Autodesk Inventor part; units mm, degrees
ref_plane "Work Plane1" through (0, 58, 0) normal (0, 1, 0) x (1, 0, 0)
ref_plane "YZ Plane" through (0, 0, 0) normal (1, 0, 0) x (0, 1, 0)
ref_plane "XZ Plane" through (0, 0, 0) normal (0, 1, 0) x (-1, 0, 0)
sketch "Sketch1" plane through (0, 0, 0) normal (0, 1, 0) x (-1, 0, 0)
  line L0 (25, 35) -> (-25, 35)
  line L1 (-25, 35) -> (-25, -35)
  line L2 (-25, -35) -> (25, -35)
  line L3 (25, -35) -> (25, 35)
  line L4 (25, 35) -> (-25, -35) construction
  line L5 (-25, 35) -> (25, -35) construction
  point P0 (0, 0)
  dimension "d0" = 50
  dimension "d1" = 70
extrude "Extrusion1" add sketch "Sketch1" along normal blind 4
sketch "Sketch2" plane through (0, 4, 0) normal (0, 1, 0) x (1, 0, 0)
  line L0 (25, -35) -> (25, 35)
  line L1 (25, 35) -> (-25, 35)
  line L2 (25, -35) -> (20, -35)
  line L3 (20, -35) -> (20, 35)
  line L4 (20, 35) -> (25, 35)
  line L5 (25, 35) -> (25, -35)
  line L6 (-25, 35) -> (-25, -35)
  line L7 (-25, -35) -> (-20, -35)
  line L8 (-20, -35) -> (-20, 35)
  line L9 (-20, 35) -> (-25, 35)
  line L10 (-25, 35) -> (-25, -35)
  point P0 (0, 0)
  dimension "d4" = 5
  dimension "d5" = 5
  dimension "d6" = 70
extrude "Extrusion2" add sketch "Sketch2" along normal blind 20
sketch "Sketch3" plane through (0, 24, 0) normal (0, 1, 0) x (1, 0, 0)
  line L0 (-25, -35) -> (25, -35)
  line L1 (25, -35) -> (25, 35)
  line L2 (-25, -35) -> (25, -35)
  line L3 (25, -35) -> (25, 35)
  line L4 (25, 35) -> (-25, 35)
  line L5 (-25, 35) -> (-25, -35)
  line L6 (-20, -20) -> (20, -20)
  line L7 (20, -20) -> (20, 20)
  line L8 (20, 20) -> (-20, 20)
  line L9 (-20, 20) -> (-20, -20)
  line L10 (-20, -20) -> (20, 20) construction
  line L11 (20, -20) -> (-20, 20) construction
  line L12 (-15.5, -29) -> (7.5, -29) construction
  line L13 (7.5, -29) -> (7.5, 29) construction
  line L14 (7.5, 29) -> (-15.5, 29) construction
  line L15 (-15.5, 29) -> (-15.5, -29) construction
  circle A0 centre (-15.5, -29) radius 1.5
  circle A1 centre (-15.5, 29) radius 1.5
  circle A2 centre (7.5, 29) radius 1.5
  circle A3 centre (7.5, -29) radius 1.5
  point P0 (0, 0)
  dimension "d9" = 40
  dimension "d10" = 40
  dimension "d13" = 23
  dimension "d14" = 58
  dimension "d15" = 6
  dimension "d16" = 4.5
  dimension "d17" = 3
  dimension "d18" = 3
  dimension "d19" = 3
  dimension "d20" = 3
extrude "Extrusion3" add sketch "Sketch3" along normal blind 4
sketch "Sketch4" plane through (-25, 0, -35) normal (-1, 0, 0) x (0, 0, 1)
  line L0 (9, 20) -> (61, 20)
  line L1 (61, 20) -> (61, 4)
  line L2 (61, 4) -> (9, 4)
  line L3 (9, 4) -> (9, 20)
  line L4 (0, 28) -> (70, 28)
  line L5 (0, 0) -> (0, 28)
  point P0 (35, 0)
  dimension "d21" = 52
  dimension "d22" = 16
  dimension "d23" = 8
  dimension "d24" = 9
extrude "Extrusion4" cut sketch "Sketch4" against normal blind 5
sketch "Sketch5" plane through (0, 28, 0) normal (0, 1, 0) x (1, 0, 0)
  line L0 (25, 35) -> (-25, 35)
  line L1 (-20, 35) -> (-20, 26)
  line L2 (-25, 35) -> (-20, 35)
  line L3 (-20, 35) -> (-20, 26)
  line L4 (-20, 26) -> (-25, 26)
  line L5 (-25, 26) -> (-25, 35)
  line L6 (-25, -35) -> (25, -35)
  line L7 (20, -20) -> (20, -35)
  line L8 (25, -35) -> (20, -35)
  line L9 (20, -35) -> (20, -26)
  line L10 (20, -26) -> (25, -26)
  line L11 (25, -26) -> (25, -35)
  line L12 (-25, 35) -> (-25, -35)
  line L13 (-20, -26) -> (-20, -35)
  line L14 (-25, -35) -> (-20, -35)
  line L15 (-20, -35) -> (-20, -26)
  line L16 (-20, -26) -> (-25, -26)
  line L17 (-25, -26) -> (-25, -35)
  line L18 (20, -35) -> (20, 35)
  line L19 (25, 35) -> (20, 35)
  line L20 (20, 35) -> (20, 26)
  line L21 (20, 26) -> (25, 26)
  line L22 (25, 26) -> (25, 35)
  point P0 (0, 0)
  dimension "d27" = 9
  dimension "d28" = 9
extrude "Extrusion5" add sketch "Sketch5" along normal blind 53 contours L22 L21 L18 L0 | L1 L4 L5 L0 | L10 L11 L6 L7 | L16 L13 L6 L12
sketch "Sketch6" plane through (0, 81, 0) normal (0, 1, 0) x (1, 0, 0)
  line L0 (-25, 35) -> (-25, -35)
  line L1 (20, -35) -> (25, -35)
  line L2 (-25, 35) -> (25, 35)
  line L3 (25, 35) -> (25, -35)
  line L4 (25, -35) -> (-25, -35)
  line L5 (-25, -35) -> (-25, 35)
  line L6 (-10, -10) -> (10, -10) construction
  line L7 (10, -10) -> (10, 10) construction
  line L8 (10, 10) -> (-10, 10) construction
  line L9 (-10, 10) -> (-10, -10) construction
  line L10 (-10, -10) -> (10, 10) construction
  line L11 (10, -10) -> (-10, 10) construction
  line L12 (-25, 25) -> (25, 25) construction
  line L13 (25, 25) -> (25, -25) construction
  line L14 (25, -25) -> (-25, -25) construction
  line L15 (-25, -25) -> (-25, 25) construction
  line L16 (-25, 25) -> (25, -25) construction
  line L17 (25, 25) -> (-25, -25) construction
  line L18 (20, 20) -> (20, -20) construction
  line L19 (-20, 20) -> (20, 20) construction
  line L20 (20, 20) -> (20, -20) construction
  line L21 (20, -20) -> (-20, -20) construction
  line L22 (-20, -20) -> (-20, 20) construction
  line L23 (-20, 20) -> (20, -20) construction
  line L24 (20, 20) -> (-20, -20) construction
  line L25 (-16, 16) -> (16, 16)
  line L26 (16, 16) -> (16, -16)
  line L27 (16, -16) -> (-16, -16)
  line L28 (-16, -16) -> (-16, 16)
  line L29 (-16, 16) -> (16, -16) construction
  line L30 (16, 16) -> (-16, -16) construction
  point P0 (0, 0)
  dimension "d31" = 20
  dimension "d32" = 20
  dimension "d33" = 50
  dimension "d34" = 50
  dimension "d35" = 40
  dimension "d36" = 40
  dimension "d37" = 32
  dimension "d38" = 32
extrude "Extrusion6" add sketch "Sketch6" along normal blind 4
sketch "Sketch7" plane through (0, 85, 0) normal (0, 1, 0) x (1, 0, 0)
  line L0 (20, 20) -> (20, -20) construction
  line L1 (-20, 20) -> (20, 20) construction
  line L2 (20, 20) -> (20, -20) construction
  line L3 (20, -20) -> (-20, -20) construction
  line L4 (-20, -20) -> (-20, 20) construction
  line L5 (-20, 20) -> (20, -20) construction
  line L6 (20, 20) -> (-20, -20) construction
  circle A0 centre (-20, 20) radius 2.5
  line L7 (-20, 20) -> (20, 20)
  circle A1 centre (20, 20) radius 2.5
  circle A2 centre (20, -20) radius 2.5
  line L8 (20, -20) -> (-20, -20)
  circle A3 centre (-20, -20) radius 2.5
  point P0 (0, 0)
  dimension "d41" = 40
  dimension "d42" = 40
  dimension "d43" = 5
  dimension "d44" = 5
  dimension "d45" = 5
  dimension "d46" = 5
extrude "Extrusion7" add sketch "Sketch7" along normal blind 8
sketch "Sketch8" plane through (25, 0, 35) normal (1, 0, 0) x (0, 0, -1)
  line L0 (15, 28) -> (55, 28)
  line L1 (9, 4) -> (61, 4)
  line L2 (15, 28) -> (55, 28)
  line L3 (55, 28) -> (55, 4)
  line L4 (55, 4) -> (15, 4)
  line L5 (15, 4) -> (15, 28)
  point P0 (15, 4)
  dimension "d53" = 40
extrude "Extrusion8" cut sketch "Sketch8" against normal blind 5
ref_plane "Work Plane1" through (0, 58, 0) normal (0, 1, 0) x (1, 0, 0)
sketch "Sketch9" plane through (0, 58, 0) normal (0, 1, 0) x (1, 0, 0)
  line L0 (-20, -26) -> (-20, -35)
  line L1 (20, -35) -> (20, -26)
  line L2 (-20, -35) -> (20, -35)
  line L3 (20, -35) -> (20, -26)
  line L4 (20, -26) -> (-20, -26)
  line L5 (-20, -26) -> (-20, -35)
  line L6 (-25, 26) -> (-20, 26)
  line L7 (25, 35) -> (-25, 35)
  line L8 (-20, 26) -> (20, 26)
  line L9 (20, 26) -> (20, 35)
  line L10 (20, 35) -> (-20, 35)
  line L11 (-20, 35) -> (-20, 26)
  circle A0 centre (-15.5, -29) radius 1.5
  circle A1 centre (-15.5, -29) radius 1.25
  circle A2 centre (7.5, -29) radius 1.5
  circle A3 centre (7.5, -29) radius 1.25
  circle A4 centre (-15.5, 29) radius 1.5
  circle A5 centre (-15.5, 29) radius 1.25
  circle A6 centre (7.5, 29) radius 1.5
  circle A7 centre (7.5, 29) radius 1.25
  point P0 (0, 0)
  point P1 (-20, 35)
extrude "Extrusion9" add sketch "Sketch9" against normal blind 4 contours L4 L1 L2 L0 | L9 L8 L11 L7
sketch "Sketch10" plane through (25, 0, 35) normal (1, 0, 0) x (0, 0, -1)
  line L0 (61, 20) -> (9, 20)
  line L1 (15, 4) -> (15, 28)
  line L2 (9, 20) -> (15, 20)
  line L3 (15, 20) -> (15, 4)
  line L4 (15, 4) -> (9, 4)
  line L5 (9, 4) -> (9, 20)
  point P0 (35, 0)
  point P1 (15, 20)
extrude "Extrusion10" cut sketch "Sketch10" against normal blind 5
properties part number "support"
Source: CAD feature listing. Evaluate the final solid. Frame: model axes, mm. A direction names the side the tool comes from. Coordinates: 2 decimals unless noted, no trailing zeros. Write each loop counter-clockwise with the first axis right and the second up, starting at its lowest first coordinate (ties: lowest second). Pieces come first, ordered by that corner, then holes. Notation, with made-up numbers: (-16, -29.75) -> (31, -29.75) arc R19 cw to (31, -22.75) -> close; hole circle Ø6 at (66, 44). An arc over 180 degrees is marked (long way). Return JSON: item names as keys, results as strings. Group by question number.
1) Section query D-D, the plane z = 9. Return loops of the section in (x, y), plus the area to 3 significant figures.
2) Section query C-C, the plane x = 4.5. Return loops of the section in (y, z), plus the area to 3 significant figures.
3) Ray query, line 1 along Y through (x, z) = (-9.5, -23.5); line 2 along Y through (x, z) = (-18, -28.5); line 3 along X through (y, z) = (55, 29). Return the intervals inside material, ascending.
4) Mould query, pull axis X, two halves, no side actions, for faces 6 (the face through (23, 20, 23)), 7 (the face through (16, 83, 0)). Classes: +X half, -X half, draft (parallel to the pull), parting line (faces both ways), or undercut.
5) Contact query for flat-ended pins moving along their axis: P1, Ø5, axis at x = 2, z = -11, coming from the +Y side; P2, Ø3.5, axis at x = 7.5, z = 29, coming from the +Y side. Output: stop coordinate, or through.
6) Set-up query: faces 1 (the face through (-23, 12, -26)), 2 (the face through (3, 26, 20)), 3 (the face through (-0.1, 54.4, -26)), 4 (the face through (-16.61, 56.03, 27.99)), 5 (the face through (-16, 83, 0)). Return all of +Z, -Z, +X, -X, +Y, -Y with unobstructed straight access to the full face (end or side cutting, diameter ignored); none if empty.
7) Section query B-B, the plane y = 7. Return loops of the section in (x, z), plus the area to 3 significant figures.
8) Section query A-A, the plane z = 29. State how many separate pieces and enclosed holes the cut face has, plus the area to 3 significant figures.
From the geometry:
{
 "1": {"outline": "(-25, 0) -> (25, 0) -> (25, 4) -> (-25, 4) -> close; (-25, 20) -> (-20, 20) -> (-20, 28) -> (-25, 28) -> close; (-25, 81) -> (-16, 81) -> (-16, 85) -> (-25, 85) -> close; (16, 81) -> (25, 81) -> (25, 85) -> (16, 85) -> close", "area": "312 mm²"},
 "2": {"outline": "(0, -35) -> (4, -35) -> (4, 35) -> (0, 35) -> close; (24, -35) -> (28, -35) -> (28, -20) -> (24, -20) -> close; (24, 20) -> (28, 20) -> (28, 35) -> (24, 35) -> close; (54, -35) -> (58, -35) -> (58, -26) -> (54, -26) -> close; (54, 26) -> (58, 26) -> (58, 35) -> (54, 35) -> close; (81, -35) -> (85, -35) -> (85, -16) -> (81, -16) -> close; (81, 16) -> (85, 16) -> (85, 35) -> (81, 35) -> close", "area": "624 mm²"},
 "3": {"line 1": "0 to 4, 24 to 28, 81 to 85", "line 2": "0 to 4, 24 to 28, 54 to 58, 81 to 85", "line 3": "-25 to -17, -14 to 6, 9 to 25"},
 "4": {"face 6": "draft", "face 7": "undercut"},
 "5": {"P1": "y = 4", "P2": "y = 85"},
 "6": {"face 1": "-X", "face 2": "+X", "face 3": "+X, -X", "face 4": "none", "face 5": "+Y"},
 "7": {"outline": "(-25, -35) -> (-20, -35) -> (-20, -26) -> (-25, -26) -> close; (-25, 26) -> (-20, 26) -> (-20, 35) -> (-25, 35) -> close; (20, -35) -> (25, -35) -> (25, -20) -> (20, -20) -> close; (20, 26) -> (25, 26) -> (25, 35) -> (20, 35) -> close", "area": "210 mm²"},
 "8": {"separate pieces": "3", "enclosed holes": "1", "area": "1,440 mm²"}
}
